Here's the drawing with two shaded views (mm, measured from the low corner). I have some questions. A direction names the side the tool comes from. Give positions to 0.01 mm unless a question says otherwise; leave off trailing zeros. Write each loop counter-clockwise with the first axis right and the second up, starting at its lowest first coordinate (ties: lowest second). Pieces come first, ordered by that corner, then holes. Notation, with made-up numbers: (-15.5, 34.25) - (38.5, 34.25) arc R23 cw to (38.5, 59.25) - close; hole circle Ø9 at (-2.5, -22.5). An arc over 180 degrees is marked (long way). Answer as CSV lines item,"result". Start each with the question number.
Q1. If I drill on line 1 along Z through (x, y) = (73.5, 7); line 2 along Z through (x, y) = (103.5, 18.5); line 3 along X through (y, z) = (10.25, 38.5), over which ranges is the centre line in solid material (lowest first)?
Q2. On a 3-axis mill with a long thin cutter (end or side, diameter ignored), from which of +Z, -Z, +X, -X, +Y, -Y can I reach the whole of each face in a straight line? I mean the marked faces 1 and 2. Say none if no direction works.
Q3. We'd pull the mould along X, two halves only. Please class the marked faces 3, 4 and 5: pulls with the +X half, pulls with the -X half, needs draft (parallel to the pull), parting line crosses it, or undercut.
Q4. Will these pins go through, and if not, where does the flat tip stop? pin 1 Ø12 at (y, z) = (8, 10) entering from +X (1 decimal); pin 2 Ø4 at (y, z) = (4.5, 13.5) entering from -X (1 decimal); pin 3 Ø12 at (x, y) = (111, 22.5) entering from +Z.
Q5. Imagine slicing it at B-B on x = 45. List the corners of the cut face in (y, z) for me (1 decimal).
Q6. Imagine slicing it at C-C on z = 18. List the corners of the cut face in (x, y) for me, and give its area (4 significant figures).
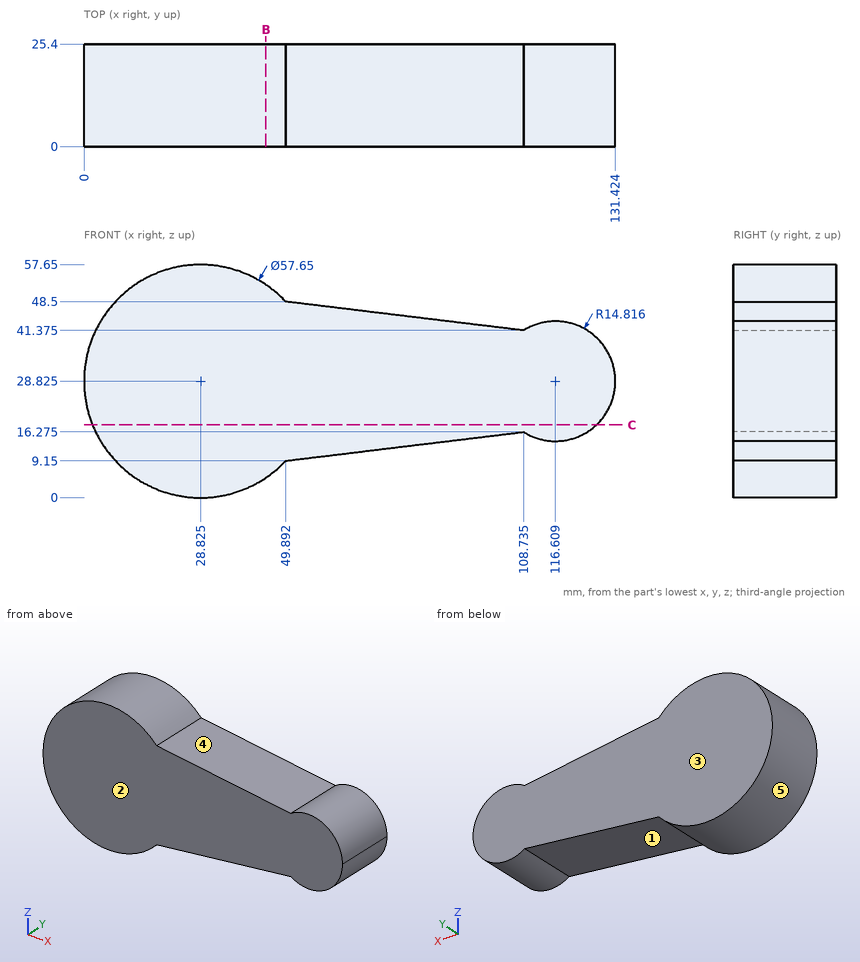
Conclusion:
1,line 1,"12.01 to 45.64"
1,line 2,"15.64 to 42.01"
1,line 3,"1.67 to 127.83"
2,face 1,"-Z, +Y, -Y"
2,face 2,"+Z, -Z, +X, -X, -Y"
3,face 3,"needs draft"
3,face 4,"undercut"
3,face 5,"parting line crosses it"
4,pin 1,"x = 124"
4,pin 2,"x = 3.3"
4,pin 3,"z = 43.64"
5,outline,"(0, 5) - (25.4, 5) - (25.4, 52.7) - (0, 52.7) - close"
6,outline,"(2.11, 0) - (126.72, 0) - (126.72, 25.4) - (2.11, 25.4) - close"
6,area,"3,165 mm^2"
